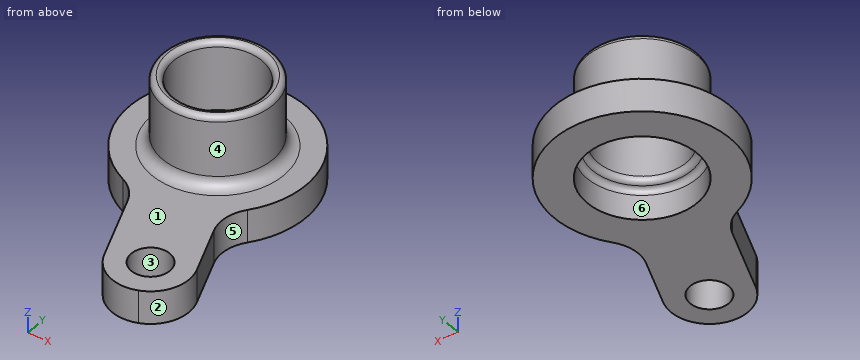
from build123d import *

# Parameters (mm, degrees)
ESQUISSE1_R             = 8
ESQUISSE1_R_2           = 5
BOSS_EXTRU_1_DEPTH      = 3
BOSS_EXTRU_2_DEPTH      = 6.5
BOSS_EXTRU_2_DEPTH_BACK = 0.25
ESQUISSE2_R             = 5
ESQUISSE2_R_2           = 4
CONG_2_R                = 0.5
ESQUISSE4_R             = 1.75
BOSS_EXTRU_4_DEPTH      = 3
CONG_3_R                = 3.5
CONG_4_R                = 1


with BuildPart() as part:
    # Esquisse1 → Boss.-Extru.1 (new body)
    with BuildSketch(Plane.XY):
        Circle(ESQUISSE1_R)
        Circle(ESQUISSE1_R_2, mode=Mode.SUBTRACT)
    extrude(amount=BOSS_EXTRU_1_DEPTH)

    # Esquisse2 → Boss.-Extru.2 (add, two sides: drawn at the far end of the back side and taken through both)
    with BuildSketch(Plane.XY.offset(3).offset(-BOSS_EXTRU_2_DEPTH_BACK)):
        Circle(ESQUISSE2_R)
        Circle(ESQUISSE2_R_2, mode=Mode.SUBTRACT)
    extrude(amount=BOSS_EXTRU_2_DEPTH + BOSS_EXTRU_2_DEPTH_BACK)

    # Congé2
    cong_2_edges = [part.edges().sort_by_distance(p)[0] for p in [
        (-5, 0, 2.75),
        (-4, 0, 2.75),
        (-4, 0, 9.5),
        (-5, 0, 9.5),
    ]]
    fillet(cong_2_edges, radius=CONG_2_R - 0.0001)  # a hair under: the kernel refuses the full size

    # Esquisse4 → Boss.-Extru.4 (add)
    with BuildSketch(Plane.XY):
        with BuildLine():
            ThreePointArc((4.877548317, -6.341097887), (1.559913464, -7.846443142), (-2.081227097, -7.724538418))
            Line((-2.081227097, -7.724538418), (2.057501229, -18.71868038))
            Line((2.057501229, -18.71868038), (8.60868038, -16.252498771))
            Line((8.60868038, -16.252498771), (4.877548317, -6.341097887))
        make_face()
        with Locations(Location((4.1, -14.21, 0), (0, 0, 180))):
            Circle(ESQUISSE4_R, mode=Mode.SUBTRACT)
    extrude(amount=BOSS_EXTRU_4_DEPTH)

    # Congé3
    cong_3_edges = [part.edges().sort_by_distance(p)[0] for p in [
        (4.877548317, -6.341097887, 1.5),
        (-2.081227097, -7.724538418, 1.5),
        (2.057501229, -18.71868038, 1.5),
        (8.60868038, -16.252498771, 1.5),
    ]]
    fillet(cong_3_edges, radius=CONG_3_R - 0.0001)  # a hair under: the kernel refuses the full size

    # Congé4
    cong_4_edges = [part.edges().sort_by_distance(p)[0] for p in [
        (-5, 0, 3),
    ]]
    fillet(cong_4_edges, radius=CONG_4_R)


solid = part.part
For this review, take the finished solid that the model builds, in its own axes (mm). Face numbers are marked on the shaded views. A direction names the side the tool comes from. Give positions to 0.01 mm unless a question says otherwise; leave off trailing zeros. Loops run counter-clockwise (first coordinate to the right, second up) from the corner with the lowest first, then second, coordinate; pieces in that order, holes last. Notation, with made-up numbers: M 77,-35.75 L 96,-35.75 A17 cw 96,-29.75 Z; hole C 48,34.5 d10. An arc over 180 degrees is marked long. Put each result on its own line as item: value. Start each with the question number.
(1) Add section D-D, the plane y = -14.21. Write out the cut boundary in (x, z), then the cut area to 3 significant figures.
(2) Machinability: for the marked faces 4, 5 and 6, which of the approach directions +Z, -Z, +X, -X, +Y, -Y give a long, thin tool a straight path to every point of the face, cutting with its end or side? Answer none if there is none.
(3) Add section C-C, the plane z = 5.25. Write out the cut boundary in (x, y), then the cut area to 3 significant figures.
(4) Wall thickness on L1, parallel to Y at x = 4.1, z = 1.6; L2, parallel to Y at x = 0, z = 6.4; L3, parallel to X at y = -14.21, z = 1.95: over which ranges is each line inside the solid? List them lowest first.
(5) For pin 1 (2 mm diameter, centred on x = 4.1, y = -14.21, fed in from +Z); pin 2 (2 mm diameter, centred on x = -4.5, y = -7, fed in from +Z), all flat-tipped, find the tip position at first contact; note any pin that passes through.
(6) The part is to be moulded in two halves that separate along X. For the marked faces 1, 2 and 3, say which applies: +X half, -X half, draft (parallel to the pull), parting line (faces both ways), or undercut.
Result:
1. outline: M 0.36,0 L 2.35,0 L 2.35,3 L 0.36,3 Z; M 5.85,0 L 7.6,0 L 7.6,3 L 5.85,3 Z
1. area: 11.2 mm^2
2. face 4: +Z
2. face 5: +Z, -Z, +X
2. face 6: -Z
3. outline: C 0,0 d10; hole C 0,0 d8
3. area: 28.3 mm^2
4. L1: y = -17.71 to -15.96, -12.46 to -2.86, 2.86 to 6.87
4. L2: y = -5 to -4, 4 to 5
4. L3: x = 0.36 to 2.35, 5.85 to 7.6
5. pin 1: passes through
5. pin 2: stops at z = 3
6. face 1: draft
6. face 2: +X half
6. face 3: undercut
